Design review of the part built by this model. Coordinates are the model's own, in mm. Face numbers are marked on the shaded views. A direction names the side the tool comes from. Coordinates: 2 decimals unless noted, no trailing zeros. Loops run counter-clockwise (first coordinate to the right, second up) from the corner with the lowest first, then second, coordinate; pieces in that order, holes last. Notation, with made-up numbers: (58, 76) -> (97, 76) arc R12 cw to (97, 80) -> close; hole circle Ø7 at (87, 43). An arc over 180 degrees is marked (long way). Use a Markdown table: item, result. Add a question column.
Q1. Take a section at A-A on y = 0. Write out the cut boundary in (x, z).
Q2. Clearance check with flat-ended pins moving along their axes: pin 1 Ø5 at (y, z) = (1, -28) entering from +X; pin 2 Ø5 at (x, y) = (-7, -9) entering from +Z; pin 3 Ø11 at (y, z) = (0.5, 9) entering from -X; pin 4 Ø8 at (y, z) = (9, -30) entering from +X. State where each tip first meets the part, or that it passes through.
Q3. For the marked faces 1, 2, 3, 4 and 5, list the 3-axis set-ups (+Z, -Z, +X, -X, +Y, -Y) from which the entire face can be reached by the end or side of a thin tool; tool diameter is ignored.
Q4. Take a section at D-D on z = -31.5. Write out the cut boundary in (x, y).
Q5. Take a section at C-C on z = -8. Write out the cut boundary in (x, y).
Q6. Take a section at B-B on z = 4.5. Write out the cut boundary in (x, y), plus the area to 3 significant figures.
Q7. For probe 1 along Z at (x, y) = (8, 4.5); probe 2 along Z at (x, y) = (-5.25, -2.25); probe 3 along Y at (x, z) = (0.5, -12), list the stretches that pass through material, from the lowest coordinate up.
from build123d import *

# Parameters (mm, degrees)
HEAD_DEPTH     = 12.954
SHANK_SKETCH_R = 6.35
SHANK_DEPTH    = 50.8
THREAD_END_W   = 31.75
THREAD_END_H   = 0.05
CHAMFER1_SIZE  = 0.79375


with BuildPart() as part:
    # Head Sketch → Head (new body)
    with BuildSketch(Plane.XY):
        Polygon((0, 10.89586975), (9.4361, 5.447934875), (9.4361, -5.447934875), (0, -10.89586975), (-9.4361, -5.447934875), (-9.4361, 5.447934875), align=None)
    extrude(amount=HEAD_DEPTH)

    # Shank Sketch → Shank (add)
    with BuildSketch(Plane.XY):
        Circle(SHANK_SKETCH_R)
    extrude(amount=-SHANK_DEPTH)

    # Sketch3 → Flange (revolve)
    with BuildSketch(Plane(origin=(0, 0, 0), x_dir=(-1, 0, 0), z_dir=(0, 1, 0))):
        with BuildLine():
            Line((-13.589, 0), (0, 0))
            Line((0, 0), (0, 4.7625))
            ThreePointArc((0, 4.7625), (-7.158083275, 3.937386416), (-13.940711322, 1.505324458))
            ThreePointArc((-13.940711322, 1.505324458), (-14.361933143, 0.613158144), (-13.589, 0))
        make_face()
    revolve(axis=Axis((0, 0, 0), (0, 0, 1)))

    # Thread End → Thread Cut (revolve, cut)
    with BuildSketch(Plane(origin=(0, 0, 0), x_dir=(0, 0, -1), z_dir=(1, 0, 0))):
        with Locations((34.925, 6.325)):
            Rectangle(THREAD_END_W, THREAD_END_H)
    revolve(axis=Axis((0, 0, -21.551935625), (0, 0, -1)), mode=Mode.SUBTRACT)

    # Chamfer1
    chamfer1_edges = [part.edges().sort_by_distance(p)[0] for p in [
        (0, -6.3, -50.8),
    ]]
    chamfer(chamfer1_edges, length=CHAMFER1_SIZE)


solid = part.part
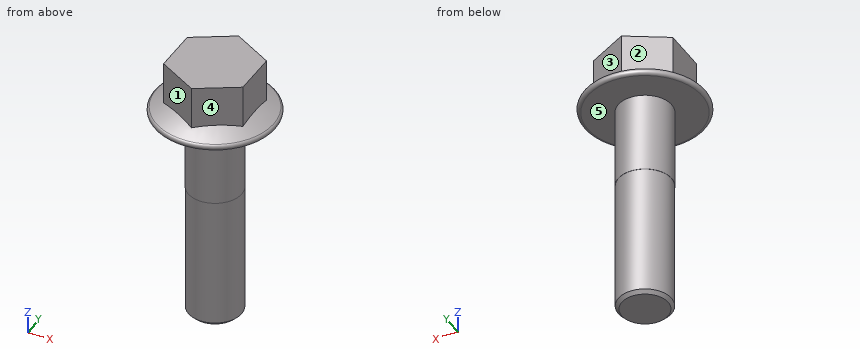
Answer list:
| question | item | result |
|---|---|---|
| 1 | outline | (-13.94, 1.51) arc R0.79 ccw to (-13.59, 0) -> (-6.35, 0) -> (-6.35, -19.05) -> (-6.3, -19.05) -> (-6.3, -50.01) -> (-5.51, -50.8) -> (5.51, -50.8) -> (6.3, -50.01) -> (6.3, -19.05) -> (6.35, -19.05) -> (6.35, 0) -> (13.59, 0) arc R0.79 ccw to (13.94, 1.51) arc R31.46 ccw to (9.44, 3.31) -> (9.44, 12.95) -> (-9.44, 12.95) -> (-9.44, 3.31) arc R31.46 ccw to start |
| 2 | pin 1 | x = 6.3 |
| 2 | pin 2 | z = 12.95 |
| 2 | pin 3 | x = -9.44 |
| 2 | pin 4 | x = 3.83 |
| 3 | face 1 | +Z, -X, -Y |
| 3 | face 2 | +Z, -X, +Y |
| 3 | face 3 | +Z, +X, +Y |
| 3 | face 4 | +Z, +X, -Y |
| 3 | face 5 | -Z |
| 4 | outline | circle Ø12.6 at (0, 0) |
| 5 | outline | circle Ø12.7 at (0, 0) |
| 6 | outline | (-9.44, -5.45) -> (0, -10.9) -> (9.44, -5.45) -> (9.44, 5.45) -> (0, 10.9) -> (-9.44, 5.45) -> close |
| 6 | area | 308 mm² |
| 7 | probe 1 | 0 to 12.95 |
| 7 | probe 2 | -50.59 to 12.95 |
| 7 | probe 3 | -6.33 to 6.33 |
